from build123d import *

# Parameters (mm, degrees)
F1_DEPTH = 2.5
F2_W     = 8
F2_H     = 10
F3_DEPTH = 8
F5_D     = 3.9
F5_DEPTH = 8
F5_TIP   = 1.1716782071


with BuildPart() as f1:
    # F0 (on Top) → F1 (new body)
    with BuildSketch(Plane.XY):
        with BuildLine():
            Line((-20.0000001545, 14.6966284215), (-58.0000001545, 14.6966284215))
            ThreePointArc((-58.0000001545, 14.6966284215), (-47.8037567712, 4.8507734158), (-44.0000001545, -8.8033715785))
            ThreePointArc((-44.0000001545, -8.8033715785), (-18.7781642386, -10.3906266976), (-1.545e-07, -27.3033715785))
            ThreePointArc((-1.545e-07, -27.3033715785), (18.7930768405, -10.4260952422), (43.9999998455, -8.8033715785))
            ThreePointArc((43.9999998455, -8.8033715785), (47.8037564623, 4.8507734158), (57.9999998455, 14.6966284215))
            Line((57.9999998455, 14.6966284215), (19.9999998455, 14.6966284215))
            ThreePointArc((19.9999998455, 14.6966284215), (14.8965569576, 6.584120609), (5.4999998455, 4.6966284215))
            Line((5.4999998455, 4.6966284215), (3.4606747963, 11.629213579))
            Line((3.4606747963, 11.629213579), (2.0776513566, 8.6966284215))
            Line((2.0776513566, 8.6966284215), (-1.9223486434, 8.6966284215))
            Line((-1.9223486434, 8.6966284215), (-3.5393252037, 11.629213579))
            Line((-3.5393252037, 11.629213579), (-5.5000001545, 4.6966284215))
            ThreePointArc((-5.5000001545, 4.6966284215), (-14.8965572665, 6.584120609), (-20.0000001545, 14.6966284215))
        make_face()
    extrude(amount=F1_DEPTH)

    # F2 (on face) → F3 (join)
    with BuildSketch(Plane.XY.offset(2.5)):
        with Locations((0.2678574529, -9.7117358875)):
            Rectangle(F2_W, F2_H)
    extrude(amount=F3_DEPTH)

    # F5
    with Locations(Plane.XZ.offset(14.7117358875)):
        with Locations((0.0262330668, 7.0685278624)):
            Hole(F5_D / 2, depth=F5_DEPTH)
            with Locations((0, 0, -(F5_DEPTH + F5_TIP / 2))):  # 118° drill point
                Cone(0, F5_D / 2, F5_TIP, mode=Mode.SUBTRACT)


solid = f1.part
Check sheet for the modelled part. Datum: model origin and axes. Units: mm. A direction names the side the tool comes from. Give positions to 0.01 mm unless a question says otherwise; leave off trailing zeros. Write each loop counter-clockwise with the first axis right and the second up, starting at its lowest first coordinate (ties: lowest second). Pieces come first, ordered by that corner, then holes. Notation, with made-up numbers: M -24.5,65.25 L 29.5,65.25 A11 ccw 29.5,71.25 Z; hole C 76,-33.5 d3. An arc over 180 degrees is marked long. Use one line per item in the form item = value.
(1) Draft check along X on faces 6 (the cylindrical face through (15.01, 6.663, 1.232)), 7 (the flat face through (-1, -1, 2.5)), 8 (the cylindrical face through (47.702, 4.678, 1.232)). Enter one of: pulls with the +X half, pulls with the -X half, needs draft (parallel to the pull), parting line crosses it, or undercut.
Answer block:
face_6 = undercut
face_7 = needs draft
face_8 = pulls with the +X half
(2) Section check C-C on y = -21. Record the boundary of the cut face in (x, z), plus the area to 3 significant figures.
Answer block:
outline = M -4.33,0 L 4.36,0 L 4.36,2.5 L -4.33,2.5 Z
area = 21.7 mm2
(3) Section check A-A on z = 1. Record the boundary of the cut face in (x, y), plus the area to 3 significant figures.
Answer block:
outline = M -58,14.7 A27 cw -44,-8.8 A38.42 cw 0,-27.3 A38.56 cw 44,-8.8 A27 cw 58,14.7 L 20,14.7 A12.15 cw 5.5,4.7 L 3.46,11.63 L 2.08,8.7 L -1.92,8.7 L -3.54,11.63 L -5.5,4.7 A12.15 cw -20,14.7 Z
area = 2,230 mm2
(4) Section check B-B on x = -24.5. Record the boundary of the cut face in (y, z).
Answer block:
outline = M -8.5,0 L 14.7,0 L 14.7,2.5 L -8.5,2.5 Z
(5) Tool access check on faces 1 (the flat face through (-2.72, 10.14, 1.23)), 2 (the cylindrical face through (0.449, -10.656, 5.165)), 3 (the cylindrical face through (-19.111, -10.252, 1.232)), 4 (the flat face through (-3.732, -10, 6)), 5 (the flat face through (0.2, -14.712, 4.7)). Record the directions out of +Z, -Z, +X, -X, +Y, -Y that give a thin tool (end or side, any length) a straight path to the whole face; none if there is none.
Answer block:
face_1 = +Z, -Z, +Y
face_2 = -Y
face_3 = +Z, -Z, -Y
face_4 = +Z, -X, +Y, -Y
face_5 = +Z, +X, -X, -Y
(6) Material ranges on line 1 along Z through (x, y) = (-39.5, 1.5); line 2 along X through (y, z) = (-6.5, 2); line 3 along Y through (x, z) = (0, 8.5), recorded low to high.
Answer block:
line_1 = 0 to 2.5
line_2 = -44.11 to 44.11
line_3 = -6.4 to -4.71
(7) Depth check by flat-ended pin: P1, Ø21, axis at x = 16, y = -2, coming from the +Z side; P2, Ø1.2, axis at x = 0.5, z = 1, coming from the +Y side; P3, Ø4, axis at x = 0, z = 7, coming from the -Y side; P4, Ø1, axis at x = 2, y = 4.5, coming from the -Z side. Enter the tip coordinate at first touch or a pass-through.
Answer block:
P1 = 2.5
P2 = 8.7
P3 = -14.71
P4 = 0
